Geometry: final body of the model. Coordinates: model frame, mm. A direction names the side the tool comes from. Coordinates: 2 decimals unless noted, no trailing zeros. Write each loop counter-clockwise with the first axis right and the second up, starting at its lowest first coordinate (ties: lowest second). Pieces come first, ordered by that corner, then holes. Notation, with made-up numbers: (-31, 25) - (-24, 25) arc R21 cw to (-24, 37) - close; hole circle Ø6 at (67, 6). An arc over 180 degrees is marked (long way). Answer as a JSON object with one key per item and string values. Group by question number.
Item 1: Section B-B on x = 45. Return loops of the section in (y, z), and give its area (3 significant figures).
Item 2: First-contact query: pin 1 Ø12 at (y, z) = (5, 22) entering from +X; pin 2 Ø10.5 at (y, z) = (-52.5, 10) entering from +X; pin 3 Ø5 at (x, z) = (28.5, 15.5) entering from -Y; pin 4 Ø6.5 at (y, z) = (-15, 12) entering from -X. Flat tips, straight axial feed; report the tip coordinate or a pass-through.
Item 3: Section C-C on y = -58. Return loops of the section in (x, z), and give its area (3 significant figures).
Item 4: Set-up query: faces 4 (the flat face through (32.434, 26, 12)), 5 (the flat face through (-16, -68.537, 12)), 6 (the flat face through (-55, 15.963, 16)), 7 (the flat face through (-27, -43.537, 12)), 8 (the flat face through (-6, -6, -3)). Return all of +Z, -Z, +X, -X, +Y, -Y with unobstructed straight access to the full face (end or side cutting, diameter ignored); none if empty.
Item 5: Section A-A on z = 5.25. State how many separate pieces and enclosed holes the cut face has, and give its area (3 significant figures).
Item 6: Mould query, pull axis X, two halves, no side actions, for faces 1 (the flat face through (-38, -49, 1.6)), 2 (the flat face through (32.434, -18, 15)), 3 (the flat face through (-53.88, -52.13, -1.48)). Classes: pulls with the +X half, pulls with the -X half, needs draft (parallel to the pull), parting line crosses it, or undercut.
Item 7: Line query: line 1 along Z through (x, y) = (-49.5, -47); line 2 along X through (y, z) = (-61.5, 14.75); line 3 along Y through (x, z) = (-48, 13.5). Output: solid intervals per line, ascending. Write a range as from..to.
```python
from build123d import *

# Parameters (mm, degrees)
F1_DEPTH  = 3
F3_DEPTH  = 25
F4_W      = 13.2
F4_H      = 14.5
F4_W_2    = 42
F4_H_2    = 21
F5_DEPTH  = 25
F6_W      = 24
F6_H      = 21
F7_DEPTH  = 25
F8_W      = 24
F8_H      = 21
F9_DEPTH  = 25
F10_W     = 24
F10_H     = 21
F11_DEPTH = 25
F12_W     = 9
F12_H     = 21
F12_W_2   = 13.2
F12_H_2   = 13.2
F13_DEPTH = 25


with BuildPart() as f1:
    # F0 (on Top) → F1 (new body)
    with BuildSketch(Plane.XY):
        Polygon((52.4343535528, 49.4626009114), (-62.0656464472, 49.4626009114), (-62.0656464472, -41.0373990886), (-45.4653799534, -63.5373990886), (33.0013521016, -63.5373990886), (52.4343535528, -41.0373990886), align=None)
    extrude(amount=-F1_DEPTH)

    # F2 (on face) → F3 (join)
    with BuildSketch(Plane.XY):
        Polygon((52.4343535528, 54.4626009114), (-62.0656464472, 54.4626009114), (-67.0656464472, 54.4626009114), (-67.0656464472, -42.682259346), (-47.9899926711, -68.5373990886), (35.2896436851, -68.5373990886), (57.4343535528, -42.8977173713), (57.4343535528, 54.4626009114), align=None)
    extrude(amount=F3_DEPTH)

    # F4 (on face) → F5 (cut)
    with BuildSketch(Plane.YZ.offset(57.4343535528)):
        with Locations((-17.7373990886, 14.955594413)):
            Rectangle(F4_W, F4_H)
        with Locations((25.8626009114, 11.9932589587)):
            Rectangle(F4_W_2, F4_H_2)
    extrude(amount=-F5_DEPTH, mode=Mode.SUBTRACT)

    # F6 (on face) → F7 (cut)
    with BuildSketch(Plane(origin=(54.1161959556, -46.7395606462, 0), x_dir=(0.6536426668, 0.7568033193, 0), z_dir=(0.7568033193, -0.6536426668, 0))):
        with Locations((-12.2025143201, 12.1)):
            Rectangle(F6_W, F6_H)
    extrude(amount=-F7_DEPTH, mode=Mode.SUBTRACT)

    # F8 (on face) → F9 (cut)
    with BuildSketch(Plane.XZ.offset(68.5373990886)):
        with Locations((-30.1374887228, 12.1)):
            Rectangle(F8_W, F8_H)
        with Locations((20.0539599173, 12.1)):
            Rectangle(F8_W, F8_H)
    extrude(amount=-F9_DEPTH, mode=Mode.SUBTRACT)

    # F10 (on face) → F11 (cut)
    with BuildSketch(Plane(origin=(-63.8179335995, -47.0842091039, 0), x_dir=(0.5936930871, -0.8046915672, 0), z_dir=(-0.8046915672, -0.5936930871, 0))):
        with Locations((12, 12.1)):
            Rectangle(F10_W, F10_H)
    extrude(amount=-F11_DEPTH, mode=Mode.SUBTRACT)

    # F12 (on face) → F13 (cut)
    with BuildSketch(Plane(origin=(-67.0656464472, 0, 0), x_dir=(0, -1, 0), z_dir=(-1, 0, 0))):
        with Locations((-36.9626009114, 12.1)):
            Rectangle(F12_W, F12_H)
        with Locations((-9.3626009114, 16)):
            Rectangle(F12_W_2, F12_H_2)
        with Locations((17.1373990886, 12.1)):
            Rectangle(F12_W_2, F12_H)
        with Locations((33.082259346, 16)):
            Rectangle(F12_W_2, F12_H_2)
    extrude(amount=-F13_DEPTH, mode=Mode.SUBTRACT)


solid = f1.part
```
Checks:
{
 "1": {"outline": "(-57.29, 0) - (-49.65, 0) - (-49.65, -3) - (49.46, -3) - (49.46, 0) - (54.46, 0) - (54.46, 25) - (-57.29, 25) - (-57.29, 22.6) - (-39.13, 22.6) - (-39.13, 1.6) - (-57.29, 1.6) - close; hole (-24.34, 7.71) - (-11.14, 7.71) - (-11.14, 22.21) - (-24.34, 22.21) - close; hole (4.86, 1.49) - (46.86, 1.49) - (46.86, 22.49) - (4.86, 22.49) - close", "area": "1,640 mm^2"},
 "2": {"pin 1": "x = 57.43", "pin 2": "x = 8.05", "pin 3": "y = -41.05", "pin 4": "x = -42.07"},
 "3": {"outline": "(-55.76, 0) - (-49.55, 0) - (-49.55, -3) - (37.78, -3) - (37.78, 0) - (44.39, 0) - (44.39, 1.6) - (8.05, 1.6) - (8.05, 22.6) - (44.39, 22.6) - (44.39, 25) - (-55.76, 25) - (-55.76, 22.6) - (-18.14, 22.6) - (-18.14, 1.6) - (-55.76, 1.6) - close", "area": "1,210 mm^2"},
 "4": {"face 4": "+X", "face 5": "+Z, -Z, +X, -X, -Y", "face 6": "-X", "face 7": "-Y", "face 8": "-Z, +X, -X, +Y, -Y"},
 "5": {"separate pieces": "3", "enclosed holes": "0", "area": "11,000 mm^2"},
 "6": {"face 1": "undercut", "face 2": "pulls with the +X half", "face 3": "pulls with the -X half"},
 "7": {"line 1": "-3..1.6, 22.6..25", "line 2": "-42.93..-42.14, -18.14..8.05, 32.05..34.18", "line 3": "-68.52..-65.24, -26.48..-23.74, -10.54..2.76, 15.96..32.46, 41.46..54.46"}
}
